from build123d import *

# Parameters (mm, degrees)
F0_R     = 2
F0_R_2   = 5
F0_W     = 15
F0_H     = 15
F1_DEPTH = 2.5
F2_R     = 5
F3_DEPTH = 5


with BuildPart() as f1:
    # F0 (on Top) → F1 (new body)
    with BuildSketch(Plane.XY):
        Polygon((0, 25), (0, 0), (3, 0), (3, 3), (6, 3), (6, 0), (10, 0), (10, 6), (16, 6), (16, 0), (22, 0), (22, 8), (30, 8), (30, 0), (50, 0), (50, 25), align=None)
        with Locations((4.25116, 7.565503)):
            Circle(F0_R, mode=Mode.SUBTRACT)
        with Locations((8, 17)):
            Circle(F0_R_2, mode=Mode.SUBTRACT)
        with Locations((40.5, 12.5)):
            Rectangle(F0_W, F0_H, mode=Mode.SUBTRACT)
    extrude(amount=F1_DEPTH)

    # F2 (on face) → F3 (join)
    with BuildSketch(Plane.XY.offset(2.5)):
        with Locations((22.548001, 17)):
            Circle(F2_R)
    extrude(amount=F3_DEPTH)


solid = f1.part
The listing builds one solid part. Answer for the finished solid, in the listing's coordinates (mm). A direction names the side the tool comes from. Give positions to 0.01 mm unless a question says otherwise; leave off trailing zeros. Write each loop counter-clockwise with the first axis right and the second up, starting at its lowest first coordinate (ties: lowest second). Pieces come first, ordered by that corner, then holes. Notation, with made-up numbers: (49.25, 27) - (105.25, 27) arc R24 cw to (105.25, 39) - close; hole circle Ø6 at (37, 27.5). An arc over 180 degrees is marked (long way). One line per question, with ' | ' between items. Start each with the question number.
1. Determine the mould class of faces 1 (the face through (19, 0, 1)), 2 (the face through (48, 12, 1)), 3 (the face through (24.855, 12.564, 4.965)) for opening direction X: +X half, -X half, draft (parallel to the pull), parting line (faces both ways), or undercut.
2. Straight lines are drawn through the part: line 1 (Y direction, x = 45.5, z = 1); line 2 (Y direction, x = 4.5, z = 0.5); line 3 (Y direction, x = 8, z = 1.7). For each, find the intervals that lie inside material, in ascending order.
3. Given P1, Ø2, axis at x = 27.5, z = 1.5, coming from the -Y side; P2, Ø2.5, axis at x = 4.25, y = 7.57, coming from the +Z side; P3, Ø11.5, axis at x = 8, y = 17, coming from the +Z side; P4, Ø3, axis at x = 13.5, z = 1.5, coming from the -Y side, each flat-ended and moving along its own axis, determine where each tip first touches the part or whether it passes through.
4. Section B-B, the plane x = 8 is taken. Determine the outline of the cut face in (y, z).
5. Section C-C, the plane y = 17 is taken. Determine the outline of the cut face in (x, z), then the cut area to 4 significant figures.
6. For faces 4 (the face through (26, 8, 1)), 5 (the face through (0, 13, 1)), 6 (the face through (33, 12, 1)), determine the directions among +Z, -Z, +X, -X, +Y, -Y from which every point of the face is accessible in a straight line to the end or side of a thin tool.
7. Section A-A, the plane y = 11 is taken. Determine the outline of the cut face in (x, z).
8. Section D-D, the plane x = 27 is taken. Determine the outline of the cut face in (y, z).
Result:
1) face 1: draft | face 2: undercut | face 3: parting line
2) line 1: y = 0 to 5, 20 to 25 | line 2: y = 3 to 5.58, 9.55 to 13.43, 20.57 to 25 | line 3: y = 0 to 12, 22 to 25
3) P1: stops at y = 8 | P2: passes through | P3: stops at z = 2.5 | P4: stops at y = 6
4) outline: (0, 0) - (12, 0) - (12, 2.5) - (0, 2.5) - close; (22, 0) - (25, 0) - (25, 2.5) - (22, 2.5) - close
5) outline: (0, 0) - (3, 0) - (3, 2.5) - (0, 2.5) - close; (13, 0) - (33, 0) - (33, 2.5) - (27.55, 2.5) - (27.55, 7.5) - (17.55, 7.5) - (17.55, 2.5) - (13, 2.5) - close; (48, 0) - (50, 0) - (50, 2.5) - (48, 2.5) - close | area: 112.5 mm2
6) face 4: +Z, -Z, -Y | face 5: +Z, -Z, -X, +Y, -Y | face 6: +Z, -Z
7) outline: (0, 0) - (33, 0) - (33, 2.5) - (0, 2.5) - close; (48, 0) - (50, 0) - (50, 2.5) - (48, 2.5) - close
8) outline: (8, 0) - (25, 0) - (25, 2.5) - (19.28, 2.5) - (19.28, 7.5) - (14.72, 7.5) - (14.72, 2.5) - (8, 2.5) - close
